```python
from build123d import *

# Parameters (mm, degrees)
SKETCH1_R           = 1.5
SKETCH1_R_2         = 2
SKETCH1_R_3         = 1
BOSS_EXTRUDE1_DEPTH = 5


with BuildPart() as part:
    # Sketch1 → Boss-Extrude1 (new body)
    with BuildSketch(Plane(origin=(0, 0, 0), x_dir=(1, 0, 0), z_dir=(0, 1, 0))):
        with BuildLine():
            Line((-8.762210389, 5.828693601), (-0.11807649, 5.998838049))
            ThreePointArc((-0.11807649, 5.998838049), (0.662554919, 5.963306212), (1.431947779, 5.82662214))
            ThreePointArc((1.431947779, 5.82662214), (13.458528139, 4.649327756), (25.539939967, 4.902597239))
            ThreePointArc((25.539939967, 4.902597239), (30.995866152, 0.235754194), (26.175572284, -5.085084233))
            ThreePointArc((26.175572284, -5.085084233), (13.230242543, -6.601805731), (0.210435347, -5.996308612))
            ThreePointArc((0.210435347, -5.996308612), (-1.508245613, -5.807339767), (-3.101676264, -5.136107899))
            ThreePointArc((-3.101676264, -5.136107899), (-6.887532568, -3.042769433), (-10.502643591, -0.666691535))
            ThreePointArc((-10.502643591, -0.666691535), (-12.074072829, 3.235238064), (-8.762210389, 5.828693601))
        make_face()
        Circle(SKETCH1_R, mode=Mode.SUBTRACT)
        with Locations((26, -0.082190865)):
            Circle(SKETCH1_R_2, mode=Mode.SUBTRACT)
        with Locations((-8.693332437, 2.329371406)):
            Circle(SKETCH1_R_3, mode=Mode.SUBTRACT)
    extrude(amount=BOSS_EXTRUDE1_DEPTH)


solid = part.part
```
Input: part model. Units: mm. Frame: model coordinates. Coordinates: 2 decimals unless noted, no trailing zeros. Write each loop counter-clockwise with the first axis right and the second up, starting at its lowest first coordinate (ties: lowest second). Pieces come first, ordered by that corner, then holes. Notation, with made-up numbers: (-19, 43.25) -> (36, 43.25) arc R17 cw to (36, 56.25) -> close; hole circle Ø7 at (37.5, 12). An arc over 180 degrees is marked (long way). Write each question's results on one line, items separated by ' | '.
Item 1: Pin query (flat end, axial travel): pin 1 Ø2 at (x, y) = (22, 2.5) entering from -Z; pin 2 Ø1.5 at (x, y) = (22, 1.5) entering from +Z; pin 3 Ø2 at (x, y) = (-7.5, 1.5) entering from +Z; pin 4 Ø2.5 at (x, z) = (0, 0) entering from -Y. Return the tip coordinate at first contact, or that it passes through.
Conclusion:
pin 1: stops at z = -4.73 | pin 2: stops at z = 5.92 | pin 3: stops at z = 3.27 | pin 4: passes through
Item 2: Section query C-C on z = 4.25. Return loops of the section in (x, y).
Conclusion:
outline: (-4.79, 0) -> (28.77, 0) -> (28.77, 5) -> (-4.79, 5) -> close
Item 3: Section query A-A on y = 2.15. Return loops of the section in (x, z).
Conclusion:
outline: (-10.5, 0.67) arc R3.5 ccw to (-8.76, -5.83) -> (-0.12, -6) arc R6 ccw to (1.43, -5.83) arc R102 cw to (25.54, -4.9) arc R5.01 ccw (long way) to (26.18, 5.09) arc R80 ccw to (0.21, 6) arc R6 ccw to (-3.1, 5.14) arc R56.66 ccw to start; hole circle Ø2 at (-8.69, -2.33); hole circle Ø3 at (0, 0); hole circle Ø4 at (26, 0.08)
Item 4: Section query B-B on x = -3.5. Return loops of the section in (y, z), plus the area to 3 significant figures.
Conclusion:
outline: (0, -5.93) -> (5, -5.93) -> (5, 4.93) -> (0, 4.93) -> close | area: 54.3 mm^2
Item 5: Material intervals for probe 1 along Z at (x, y) = (0, 4.4); probe 2 along X at (y, z) = (0.7, 1.25); probe 3 along Z at (x, y) = (25.5, 1.25), sorted ascending.
Conclusion:
probe 1: z = -6 to -1.5, 1.5 to 6 | probe 2: x = -9.67 to -0.83, 0.83 to 24.38, 27.62 to 30.87 | probe 3: z = -4.9 to -1.85, 2.02 to 5.22
Item 6: Mould query, pull axis X, two halves, no side actions, for faces 1 (the cylindrical face through (-12.09, 2.46, -3.17)), 2 (the flat face through (10, 0, 0)), 3 (the cylindrical face through (-1.5, 2.46, -0.07)). Classes: +X half, -X half, draft (parallel to the pull), parting line (faces both ways), or undercut.
Conclusion:
face 1: -X half | face 2: draft | face 3: undercut
